from build123d import *

# Parameters (mm, degrees)
SKETCH1_R           = 3
BOSS_EXTRUDE2_DEPTH = 4
SKETCH1_7_R         = 3
BOSS_EXTRUDE3_DEPTH = 21
CHAMFER2_SIZE       = 0.75
SKETCH3_OUTSIDE_W   = 93.502
SKETCH3_OUTSIDE_H   = 91.722
SKETCH3_OUTSIDE_R   = 5.75
CUT_EXTRUDE1_DEPTH  = 21
CUT_EXTRUDE1_DRAFT  = -60


with BuildPart() as part:
    # Sketch1 → Boss-Extrude2 (new body)
    # profile 1 of 2: a face of its own
    with BuildSketch(Plane(origin=(0, 0, 0), x_dir=(1, 0, 0), z_dir=(0, 1, 0))):
        Polygon((-3.319764048, -5.75), (3.319764048, -5.75), (6.639528096, 0), (3.319764048, 5.75), (-3.319764048, 5.75), (-6.639528096, 0), align=None)
        Circle(SKETCH1_R, mode=Mode.SUBTRACT)
    # profile 2 of 2: a face of its own
    with BuildSketch(Plane(origin=(0, 0, 0), x_dir=(1, 0, 0), z_dir=(0, 1, 0))):
        Circle(SKETCH1_R)
    extrude(amount=-BOSS_EXTRUDE2_DEPTH)

    # Sketch1_7 → Boss-Extrude3 (add)
    with BuildSketch(Plane(origin=(0, 0, 0), x_dir=(1, 0, 0), z_dir=(0, 1, 0))):
        with Locations(Location((0, 0, 0), (0, 0, 270))):
            Circle(SKETCH1_7_R)
    extrude(amount=-BOSS_EXTRUDE3_DEPTH)

    # Chamfer2
    chamfer2_edges = [part.edges().sort_by_distance(p)[0] for p in [
        (0, -21, -3),
    ]]
    chamfer(chamfer2_edges, length=CHAMFER2_SIZE)


with BuildPart() as cut_extrude1_tool:
    # Sketch3 outside → Cut-Extrude1 (with draft: the straight prism first)
    with BuildSketch(Plane(origin=(0, 0, 0), x_dir=(1, 0, 0), z_dir=(0, 1, 0))):
        Rectangle(SKETCH3_OUTSIDE_W, SKETCH3_OUTSIDE_H)
        Circle(SKETCH3_OUTSIDE_R, mode=Mode.SUBTRACT)
    extrude(amount=-CUT_EXTRUDE1_DEPTH)
    # Cut-Extrude1: the draft: its side faces are tilted about the plane it starts from
    cut_extrude1_sides = [cut_extrude1_tool.faces().sort_by_distance(p)[0] for p in [
        (0, -10.5, 45.861),
        (46.751, -10.5, 0),
        (0, -10.5, -45.861),
        (-46.751, -10.5, 0),
        (-5.75, -10.5, 0),
    ]]
    draft(cut_extrude1_sides, Plane(origin=(0, 0, 0), x_dir=(1, 0, 0), z_dir=(0, 1, 0)), CUT_EXTRUDE1_DRAFT)


with BuildPart() as part_1:
    add(part.part)

    # Cut-Extrude1: cut by cut_extrude1_tool
    add(cut_extrude1_tool.part, mode=Mode.SUBTRACT)


solid = part_1.part
Source: CAD feature listing. Evaluate the final solid. Frame: model axes, mm. A direction names the side the tool comes from. Coordinates: 2 decimals unless noted, no trailing zeros. Write each loop counter-clockwise with the first axis right and the second up, starting at its lowest first coordinate (ties: lowest second). Pieces come first, ordered by that corner, then holes. Notation, with made-up numbers: M 62.25,35 L 68.25,35 A18 cw 68.25,70 Z; hole C -29.75,71.25 d4. An arc over 180 degrees is marked long. Use a Markdown table: item, result.
1) Reachability of faces 1 (the cylindrical face through (0.9, -12.01, 2.86)), 2 (the flat face through (0, 0, 0)) from +Z, -Z, +X, -X, +Y, -Y: full face, straight path, thin tool, end or side. Return the list, or none.
Conclusion:
| item | result |
|---|---|
| face 1 | -Y |
| face 2 | +Z, -Z, +X, -X, +Y |
2) Section A-A, the plane y = -18.5. Output: boundary loops of the cut face in (x, z), then the cut area to 3 significant figures.
Conclusion:
| item | result |
|---|---|
| outline | C 0,0 d6 |
| area | 28.3 mm^2 |
3) First-contact query: pin 1 Ø2 at (x, z) = (-4.5, -4) entering from -Y; pin 2 Ø1.5 at (y, z) = (-3.5, -4.5) entering from +X; pin 3 Ø2 at (y, z) = (-15.5, 0.5) entering from -X. Flat tips, straight axial feed; report the tip coordinate or a pass-through.
Conclusion:
| item | result |
|---|---|
| pin 1 | stops at y = -4 |
| pin 2 | stops at x = 4.47 |
| pin 3 | stops at x = -3 |
4) Ray query, L1, parallel to Y at x = 5, z = -1; L2, parallel to X at y = -15, z = 2; L3, parallel to X at y = -5.75, z = -2.25. Return the intervals inside material, ascending.
Conclusion:
| item | result |
|---|---|
| L1 | y = -4 to 0 |
| L2 | x = -2.24 to 2.24 |
| L3 | x = -1.98 to 1.98 |
